Drawing for the job (mm, zero at the part's lowest x, y, z). Coordinates: 2 decimals unless noted, no trailing zeros. Loops run counter-clockwise (first coordinate to the right, second up) from the corner with the lowest first, then second, coordinate; pieces in that order, holes last. Notation, with made-up numbers: (30.5, -9) - (81.5, -9) arc R17 ccw to (81.5, 2) - close; hole circle Ø11 at (65.5, 51.5). An arc over 180 degrees is marked (long way). Put each result on its own line as item: value.
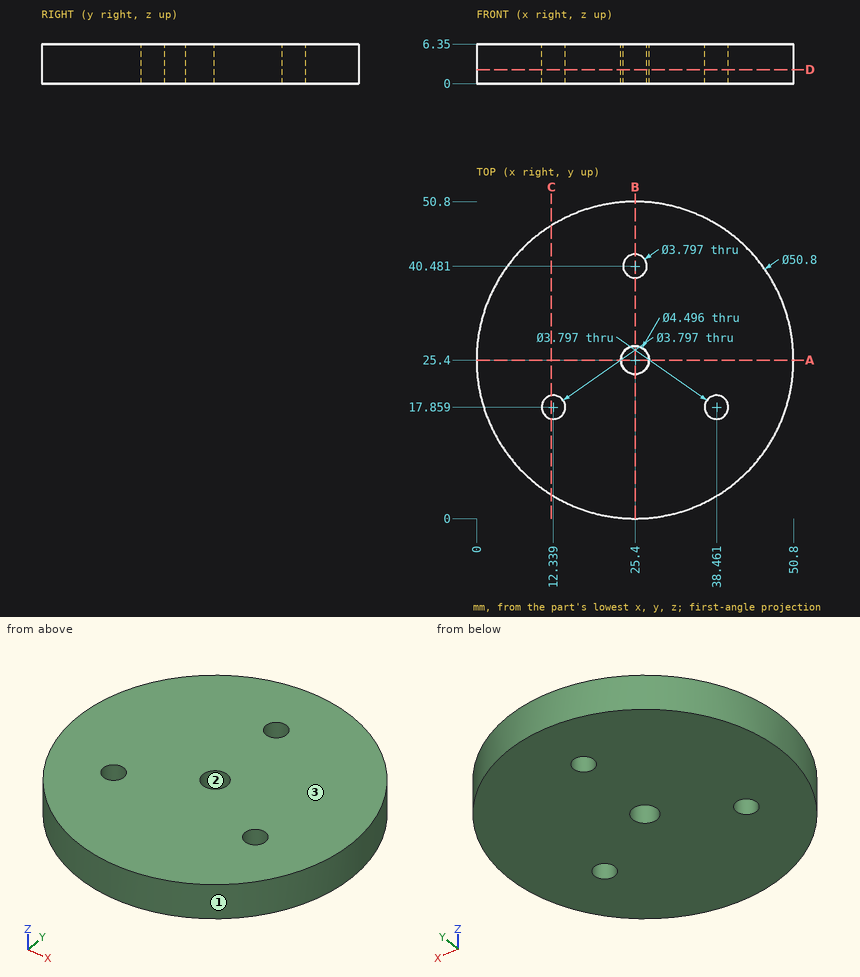
Q1. Wall check: L1, parallel to Y at x = 25.4, z = 5; L2, parallel to X at y = 18.5, z = 2.25 (1 decimal); L3, parallel to X at y = 19, z = 5.5. Give the ranges that are in metal, low to high. Write a range as from..to.
Determined:
L1: 0..23.15, 27.65..38.58, 42.38..50.8
L2: 1..10.6, 14.1..36.7, 40.2..49.8
L3: 0.82..10.82, 13.86..36.94, 39.98..49.98
Q2. Slice it at A-A, the plane y = 25.4. Give the cut face in (x, z), then the cut area to 3 significant figures.
Determined:
outline: (0, 0) - (23.15, 0) - (23.15, 6.35) - (0, 6.35) - close; (27.65, 0) - (50.8, 0) - (50.8, 6.35) - (27.65, 6.35) - close
area: 294 mm2
Q3. Slice it at B-B, the plane x = 25.4. Give the cut face in (y, z).
Determined:
outline: (0, 0) - (23.15, 0) - (23.15, 6.35) - (0, 6.35) - close; (27.65, 0) - (38.58, 0) - (38.58, 6.35) - (27.65, 6.35) - close; (42.38, 0) - (50.8, 0) - (50.8, 6.35) - (42.38, 6.35) - close
Q4. Slice it at D-D, the plane z = 2.25. Give the cut face in (x, y) (1 decimal).
Determined:
outline: circle Ø50.8 at (25.4, 25.4); hole circle Ø3.8 at (12.3, 17.9); hole circle Ø4.5 at (25.4, 25.4); hole circle Ø3.8 at (25.4, 40.5); hole circle Ø3.8 at (38.5, 17.9)
Q5. Slice it at C-C, the plane x = 12. Give the cut face in (y, z), then the cut area to 3 significant figures.
Determined:
outline: (3.82, 0) - (15.99, 0) - (15.99, 6.35) - (3.82, 6.35) - close; (19.73, 0) - (46.98, 0) - (46.98, 6.35) - (19.73, 6.35) - close
area: 250 mm2
Q6. Mould opens along Y. For the marked faces 1, 2 and 3 say: +Y half, -Y half, draft (parallel to the pull), parting line (faces both ways), or undercut.
Determined:
face 1: parting line
face 2: undercut
face 3: draft
Q7. Pin check, flat tip, straight feed: pin 1 Ø1.5 at (x, z) = (15.5, 4.5) entering from +Y (1 decimal). Stop position of the tip, or through.
Determined:
pin 1: y = 49.1
